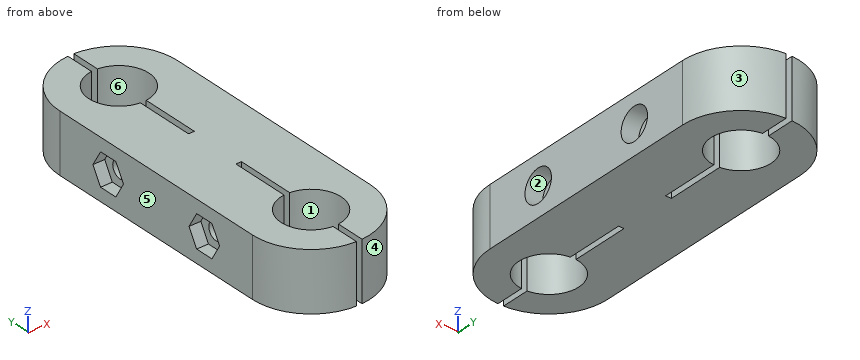
```python
from build123d import *

# Parameters (mm, degrees)
F0_R     = 5.1
F1_DEPTH = 10
F2_R     = 1.5
F3_DEPTH = 25
F5_DEPTH = 25
F6_R     = 2.75
F6_R_2   = 1.5
F7_DEPTH = 3
F8_R     = 1.5
F9_DEPTH = 2


# Not quite as in the source:
# - a feature names something its author has since deleted; it is built from what else it names


with BuildPart() as f1:
    # F0 (on Top) → F1 (new body)
    with BuildSketch(Plane.XY):
        with BuildLine():
            ThreePointArc((-10, 0), (0, -10), (10, 0))
            ThreePointArc((10, 0), (0, 10), (-10, 0))
        make_face()
        Circle(F0_R, mode=Mode.SUBTRACT)
        with BuildLine():
            Line((10, -40), (10, 0))
            ThreePointArc((10, 0), (0, -10), (-10, 0))
            Line((-10, 0), (-10, -40))
            ThreePointArc((-10, -40), (0, -30), (10, -40))
        make_face()
        with BuildLine():
            ThreePointArc((-10, -40), (0, -50), (10, -40))
            ThreePointArc((10, -40), (0, -30), (-10, -40))
        make_face()
        with Locations((0, -40)):
            Circle(F0_R, mode=Mode.SUBTRACT)
    extrude(amount=F1_DEPTH)

    # F2 (on face) → F3 (cut)
    with BuildSketch(Plane.YZ.offset(10)):
        with Locations((-30, 5)):
            Circle(F2_R)
        with Locations((-10, 5)):
            Circle(F2_R)
    extrude(amount=-F3_DEPTH, mode=Mode.SUBTRACT)

    # F4 (on face) → F5 (cut)
    with BuildSketch(Plane.XY.offset(10)):
        with BuildLine():
            ThreePointArc((0.5, 9.9874921777), (0, 10), (-0.5, 9.9874921777))
            Line((-0.5, 9.9874921777), (-0.5, 5.0754310162))
            ThreePointArc((-0.5, 5.0754310162), (0, 5.1), (0.5, 5.0754310162))
            Line((0.5, 5.0754310162), (0.5, 9.9874921777))
        make_face()
        with BuildLine():
            ThreePointArc((0.5, -5.0754310162), (0, -5.1), (-0.5, -5.0754310162))
            Line((-0.5, -5.0754310162), (-0.5, -15.1))
            Line((-0.5, -15.1), (0.5, -15.1))
            Line((0.5, -15.1), (0.5, -5.0754310162))
        make_face()
        with BuildLine():
            Line((-0.439394009, -45.0810365975), (-0.439394009, -49.9903419814))
            ThreePointArc((-0.439394009, -49.9903419814), (0.0303364777, -49.9999539848), (0.5, -49.9874921777))
            Line((0.5, -49.9874921777), (0.5, -45.0754310162))
            ThreePointArc((0.5, -45.0754310162), (0.0304323376, -45.0999092024), (-0.439394009, -45.0810365975))
        make_face()
        with BuildLine():
            Line((-0.439394009, -24.9), (-0.439394009, -34.9189634025))
            ThreePointArc((-0.439394009, -34.9189634025), (0.0304323376, -34.9000907976), (0.5, -34.9245689838))
            Line((0.5, -34.9245689838), (0.5, -24.9))
            Line((0.5, -24.9), (-0.439394009, -24.9))
        make_face()
    extrude(amount=-F5_DEPTH, mode=Mode.SUBTRACT)

    # F6 (on face) → F7 (cut)
    with BuildSketch(Plane.YZ.offset(10)):
        with Locations((-30, 5)):
            Circle(F6_R)
        with Locations((-30, 5)):
            Circle(F6_R_2, mode=Mode.SUBTRACT)
        with Locations((-10, 5)):
            Circle(F6_R)
        with Locations((-10, 5)):
            Circle(F6_R_2, mode=Mode.SUBTRACT)
    extrude(amount=-F7_DEPTH, mode=Mode.SUBTRACT)

    # F8 (on face) → F9 (cut)
    with BuildSketch(Plane(origin=(-10, 0, 0), x_dir=(0, -1, 0), z_dir=(-1, 0, 0))):
        Polygon((8.4122867597, 2.25), (11.5877132403, 2.25), (13.1754264805, 5), (11.5877132403, 7.75), (8.4122867597, 7.75), (6.8245735195, 5), align=None)
        with Locations((10, 5)):
            Circle(F8_R, mode=Mode.SUBTRACT)
        Polygon((28.4122867597, 2.25), (31.5877132403, 2.25), (33.1754264805, 5), (31.5877132403, 7.75), (28.4122867597, 7.75), (26.8245735195, 5), align=None)
        with Locations((30, 5)):
            Circle(F8_R, mode=Mode.SUBTRACT)
    extrude(amount=-F9_DEPTH, mode=Mode.SUBTRACT)


solid = f1.part
```
Read the model definition and answer for the solid it produces. Units are mm, in the model's axes. Face numbers are marked on the shaded views. A direction names the side the tool comes from. Coordinates: 2 decimals unless noted, no trailing zeros. Loops run counter-clockwise (first coordinate to the right, second up) from the corner with the lowest first, then second, coordinate; pieces in that order, holes last.
(1) Flat-ended cylindrical pins translate along their axes: pin 1 Ø5 at (x, y) = (-5, -42.5) entering from -Z; pin 2 Ø0.8 at (x, z) = (0, 7) entering from -Y; pin 3 Ø4.5 at (y, z) = (-10, 5) entering from +X; pin 4 Ø4.5 at (y, z) = (-10, 5) entering from -X. Find the tip coordinate at first contact, or state that the pin passes through.
Solution:
pin 1: stops at z = 0
pin 2: stops at y = -24.9
pin 3: stops at x = 7
pin 4: stops at x = -8
(2) The part is cut by section A-A (y = -14.5). Determine the outline of the cut face in (x, z), and give its area (3 significant figures).
Solution:
outline: (-10, 0) - (-0.5, 0) - (-0.5, 10) - (-10, 10) - close; (0.5, 0) - (10, 0) - (10, 10) - (0.5, 10) - close
area: 190 mm2
(3) The mould has two halves that part along X. Classify the marked faces 4, 5 and 6: released by +X, released by -X, zero draft, split by the parting line, or undercut.
Solution:
face 4: released by +X
face 5: released by -X
face 6: undercut
(4) Consider line 1 along X through (y, z) = (-25, 9.75); line 2 along X through (y, z) = (-39.5, 2.5); line 3 along Y through (x, z) = (-7.25, 3.75). Determine where each line is inside the solid, lowest interval first.
Solution:
line 1: x = -10 to -0.44, 0.5 to 10
line 2: x = -10 to -5.08, 5.08 to 10
line 3: y = -46.89 to -30.83, -29.17 to -10.83, -9.17 to 6.89
(5) A tool of negligible diameter and unlimited length cuts with its end or side. For the marked faces 1, 2 and 3, from which of +Z, -Z, +X, -X, +Y, -Y can it reach the whole face along a straight path? Write none if from no direction.
Solution:
face 1: +Z, -Z
face 2: +X
face 3: +Z, -Z, +X, +Y
(6) The part is cut by section C-C (z = 9). Determine the outline of the cut face in (x, y), and give its area (3 significant figures).
Solution:
outline: (-10, -40) arc R10 ccw to (-0.44, -49.99) - (-0.44, -45.08) arc R5.1 cw to (-0.44, -34.92) - (-0.44, -24.9) - (0.5, -24.9) - (0.5, -34.92) arc R5.1 cw to (0.5, -45.08) - (0.5, -49.99) arc R10 ccw to (10, -40) - (10, 0) arc R10 ccw to (0.5, 9.99) - (0.5, 5.08) arc R5.1 cw to (0.5, -5.08) - (0.5, -15.1) - (-0.5, -15.1) - (-0.5, -5.08) arc R5.1 cw to (-0.5, 5.08) - (-0.5, 9.99) arc R10 ccw to (-10, 0) - close
area: 922 mm2
(7) The part is cut by section B-B (y = -30). Determine the outline of the cut face in (x, z), and give its area (3 significant figures).
Solution:
outline: (-10, 0) - (-0.44, 0) - (-0.44, 3.5) - (-8, 3.5) - (-8, 2.25) - (-10, 2.25) - close; (-10, 7.75) - (-8, 7.75) - (-8, 6.5) - (-0.44, 6.5) - (-0.44, 10) - (-10, 10) - close; (0.5, 0) - (10, 0) - (10, 2.25) - (7, 2.25) - (7, 3.5) - (0.5, 3.5) - close; (0.5, 6.5) - (7, 6.5) - (7, 7.75) - (10, 7.75) - (10, 10) - (0.5, 10) - close
area: 121 mm2
